Read the model definition and answer for the solid it produces. Units are mm, in the model's axes. A direction names the side the tool comes from. Give positions to 0.01 mm unless a question says otherwise; leave off trailing zeros. Order: outer loops, then holes, each group sorted by start corner. A loop starts at its lowest first (then second) coordinate and runs counter-clockwise, first axis right, second up. Notation, with made-up numbers: M 20,-18.75 L 45,-18.75 A31 cw 45,7.25 Z; hole C 56.25,10.25 d5. An arc over 180 degrees is marked long. One line per item, written item: value. Start each with the question number.
from build123d import *

# Parameters (mm, degrees)
SKETCH1_R           = 2.5
SKETCH1_R_2         = 4
SKETCH1_W           = 50
SKETCH1_H           = 25
BOSS_EXTRUDE1_DEPTH = 5


with BuildPart() as part:
    # Sketch1 → Boss-Extrude1 (new body)
    with BuildSketch(Plane.XY):
        with BuildLine():
            Line((0, 27.5), (-199.858795136, 19.985879514))
            ThreePointArc((-199.858795136, 19.985879514), (-219.107383088, 0), (-199.858795136, -19.985879514))
            Line((-199.858795136, -19.985879514), (0, -27.5))
            ThreePointArc((0, -27.5), (27.5, 0), (0, 27.5))
        make_face()
        with Locations((-15, -15)):
            Circle(SKETCH1_R, mode=Mode.SUBTRACT)
        with Locations((15, 15)):
            Circle(SKETCH1_R, mode=Mode.SUBTRACT)
        with Locations((15, -15)):
            Circle(SKETCH1_R, mode=Mode.SUBTRACT)
        with Locations((-15, 15)):
            Circle(SKETCH1_R, mode=Mode.SUBTRACT)
        Circle(SKETCH1_R_2, mode=Mode.SUBTRACT)
        with Locations((-199.107383088, 0)):
            Circle(SKETCH1_R_2, mode=Mode.SUBTRACT)
        with Locations((-154.107383088, 0)):
            Rectangle(SKETCH1_W, SKETCH1_H, mode=Mode.SUBTRACT)
    extrude(amount=BOSS_EXTRUDE1_DEPTH)


solid = part.part
Q1. Find section B-B, the plane y = 0. Give the vertices of the cut face in (x, z).
Q2. Find section D-D, the plane y = 15. Give the vertices of the cut face in (x, z).
Q3. Find section A-A, the plane x = 15. Give the vertices of the cut face in (y, z).
Q4. Determine the mould class of faces 1 (the cylindrical face through (27.493, -0.605, 2.465)), 2 (the flat face through (-154, -12.5, 2)), 3 (the flat face through (-98, 0, 0)), 4 (the flat face through (-101.33, -23.69, 2.46)) for opening direction X: released by +X, released by -X, zero draft, split by the parting line, or undercut.
Q5. Consider probe 1 along Y at (x, z) = (-15, 1.35); probe 2 along X at (y, z) = (1.5, 4.35); probe 3 along X at (y, z) = (-3, 1.7). Determine where each line is inside the solid, lowest interval first.
Q6. A tool of negligible diameter and unlimited length cuts with its end or side. For faces 5 (the flat face through (-98, 0, 5)), 6 (the flat face through (-154, 12.5, 2)), from which of +Z, -Z, +X, -X, +Y, -Y can it reach the whole face along a straight path? Write none if from no direction.
Q7. Find section C-C, the plane z = 4.25. Give the vertices of the cut face in (x, y).
Q8. Each of these flat-tipped pins is pushed along its axis until it touches: pin 1 (1.5 mm diameter, centred on x = -157.5, z = 2, fed in from -Y); pin 2 (1.5 mm diameter, centred on y = -1, z = 2.5, fed in from +X); pin 3 (2.5 mm diameter, centred on x = -164.5, z = 2, fed in from +Y). Where does it stop, or does it pass through?
Evaluation:
1. outline: M -219.11,0 L -203.11,0 L -203.11,5 L -219.11,5 Z; M -195.11,0 L -179.11,0 L -179.11,5 L -195.11,5 Z; M -129.11,0 L -4,0 L -4,5 L -129.11,5 Z; M 4,0 L 27.5,0 L 27.5,5 L 4,5 Z
2. outline: M -212.34,0 L -17.5,0 L -17.5,5 L -212.34,5 Z; M -12.5,0 L 12.5,0 L 12.5,5 L -12.5,5 Z; M 17.5,0 L 23.05,0 L 23.05,5 L 17.5,5 Z
3. outline: M -23.05,0 L -17.5,0 L -17.5,5 L -23.05,5 Z; M -12.5,0 L 12.5,0 L 12.5,5 L -12.5,5 Z; M 17.5,0 L 23.05,0 L 23.05,5 L 17.5,5 Z
4. face 1: released by +X
4. face 2: undercut
4. face 3: zero draft
4. face 4: released by -X
5. probe 1: -26.94 to -17.5, -12.5 to 12.5, 17.5 to 26.94
5. probe 2: -219.05 to -202.82, -195.4 to -179.11, -129.11 to -3.71, 3.71 to 27.46
5. probe 3: -218.88 to -201.75, -196.46 to -179.11, -129.11 to -2.65, 2.65 to 27.34
6. face 5: +Z, +X, -X, +Y, -Y
6. face 6: +Z, -Z
7. outline: M -199.86,-19.99 L 0,-27.5 A27.5 ccw 0,27.5 L -199.86,19.99 A20 ccw Z; hole C -199.11,0 d8; hole M -179.11,-12.5 L -129.11,-12.5 L -129.11,12.5 L -179.11,12.5 Z; hole C -15,-15 d5; hole C -15,15 d5; hole C 0,0 d8; hole C 15,-15 d5; hole C 15,15 d5
8. pin 1: y = -21.61
8. pin 2: x = 27.5
8. pin 3: y = 21.36
